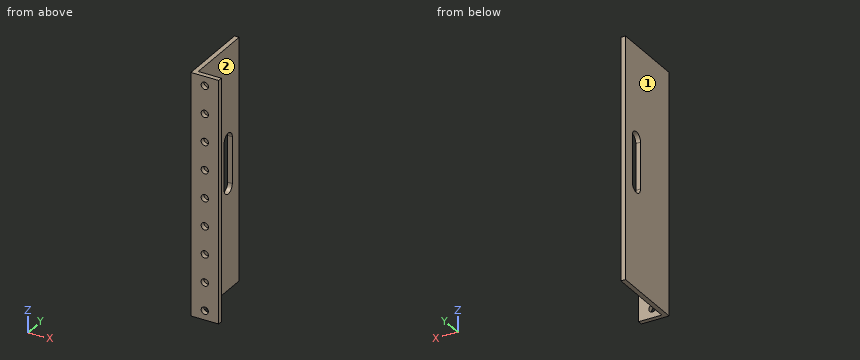
```python
from build123d import *

# Parameters (mm, degrees)
SKETCH3_W           = 3.175
SKETCH3_H           = 47.625
SKETCH3_H_2         = 3.175
SKETCH3_W_2         = 15.875
BOSS_EXTRUDE1_DEPTH = 165.1
SKETCH4_R           = 2.4892
CUT_EXTRUDE1_DEPTH  = 165.1
CUT_EXTRUDE2_DEPTH  = 165.1


with BuildPart() as part:
    # Sketch3 → Boss-Extrude1 (new body)
    with BuildSketch(Plane.XY):
        with Locations((1.5875, 26.9875)):
            Rectangle(SKETCH3_W, SKETCH3_H)
        with Locations((1.5875, 1.5875)):
            Rectangle(SKETCH3_W, SKETCH3_H_2)
        with Locations((11.1125, 1.5875)):
            Rectangle(SKETCH3_W_2, SKETCH3_H_2)
    extrude(amount=BOSS_EXTRUDE1_DEPTH)

    # Sketch4 → Cut-Extrude1 (cut)
    with BuildSketch(Plane(origin=(0, 3.175, 0), x_dir=(1, 0, 0), z_dir=(0, 1, 0))):
        with Locations(Location((9.525, -6.35, 0), (0, 0, 270))):
            Circle(SKETCH4_R)
        with Locations(Location((9.525, -25.4, 0), (0, 0, 270))):
            Circle(SKETCH4_R)
        with Locations(Location((9.525, -44.45, 0), (0, 0, 270))):
            Circle(SKETCH4_R)
        with Locations(Location((9.525, -63.5, 0), (0, 0, 270))):
            Circle(SKETCH4_R)
        with Locations(Location((9.525, -82.55, 0), (0, 0, 270))):
            Circle(SKETCH4_R)
        with Locations(Location((9.525, -101.6, 0), (0, 0, 270))):
            Circle(SKETCH4_R)
        with Locations(Location((9.525, -120.65, 0), (0, 0, 270))):
            Circle(SKETCH4_R)
        with Locations(Location((9.525, -139.7, 0), (0, 0, 270))):
            Circle(SKETCH4_R)
        with Locations(Location((9.525, -158.75, 0), (0, 0, 270))):
            Circle(SKETCH4_R)
    extrude(amount=-CUT_EXTRUDE1_DEPTH, mode=Mode.SUBTRACT)

    # Sketch5 → Cut-Extrude2 (cut)
    with BuildSketch(Plane.ZY):
        with BuildLine():
            Line((69.85, 42.8625), (101.6, 42.8625))
            ThreePointArc((101.6, 42.8625), (106.3625, 38.1), (101.6, 33.3375))
            Line((101.6, 33.3375), (69.85, 33.3375))
            ThreePointArc((69.85, 33.3375), (65.0875, 38.1), (69.85, 42.8625))
        make_face()
    extrude(amount=-CUT_EXTRUDE2_DEPTH, mode=Mode.SUBTRACT)


solid = part.part
```
The listing builds one solid part. Answer for the finished solid, in the listing's coordinates (mm). Face numbers are marked on the shaded views. A direction names the side the tool comes from. Coordinates: 2 decimals unless noted, no trailing zeros. Loops run counter-clockwise (first coordinate to the right, second up) from the corner with the lowest first, then second, coordinate; pieces in that order, holes last. Notation, with made-up numbers: (-23.5, 13.25) -> (35.5, 13.25) arc R15 cw to (35.5, 39.25) -> close; hole circle Ø6 at (-27.75, 30). An arc over 180 degrees is marked (long way). Use one line per item in the form item = value. Start each with the question number.
Item 1: Consider L1, parallel to X at y = 1.4, z = 101.6; L2, parallel to X at y = 22, z = 90 (3 decimals). Determine where each line is inside the solid, lowest interval first. Write a range as [from, to].
Item 2: The part is cut by section B-B on y = 38.1. Determine the outline of the cut face in (x, z) (1 decimal), then the cut area to 3 significant figures.
Item 3: The part is cut by section C-C on z = 82.55. Count the separate pieces of the cut face and the enclosed holes in it, then the cut area to 3 significant figures.
Item 4: The part is cut by section A-A on z = 44.45. Determine the outline of the cut face in (x, y) (3 decimals), then the cut area to 3 significant figures.
Item 5: A tool of negligible diameter and unlimited length cuts with its end or side. For the marked faces 1 and 2, from which of +Z, -Z, +X, -X, +Y, -Y can it reach the whole face along a straight path? Write none if from no direction.
Item 6: Flat-ended cylindrical pins translate along their axes: pin 1 Ø4 at (y, z) = (21, 50) entering from +X (3 decimals); pin 2 Ø10 at (x, z) = (10.5, 91) entering from +Y (3 decimals); pin 3 Ø4 at (x, z) = (9.525, 63.5) entering from +Y. Find the tip coordinate at first contact, or state that the pin passes through.
Item 7: The part is cut by section D-D on y = 26.5. Determine the outline of the cut face in (x, z) (3 decimals).
Answer key:
q1.L1 = [0, 7.04], [12.01, 19.05]
q1.L2 = [0, 3.175]
q2.outline = (0, 0) -> (3.2, 0) -> (3.2, 65.1) -> (0, 65.1) -> close; (0, 106.4) -> (3.2, 106.4) -> (3.2, 165.1) -> (0, 165.1) -> close
q2.area = 393 mm2
q3.separate_pieces = 3
q3.enclosed_holes = 0
q3.area = 166 mm2
q4.outline = (0, 0) -> (7.036, 0) -> (7.036, 3.175) -> (3.175, 3.175) -> (3.175, 50.8) -> (0, 50.8) -> close; (12.014, 0) -> (19.05, 0) -> (19.05, 3.175) -> (12.014, 3.175) -> close
q4.area = 196 mm2
q5.face_1 = +Z, -Z, -X, +Y, -Y
q5.face_2 = +Z, -Z, +X, +Y
q6.pin_1 = 3.175
q6.pin_2 = 3.175
q6.pin_3 = through
q7.outline = (0, 0) -> (3.175, 0) -> (3.175, 165.1) -> (0, 165.1) -> close
